Autodesk Inventor part; units mm, degrees
ref_plane "YZ Plane" through (0, 0, 0) normal (1, 0, 0) x (0, 1, 0)
ref_plane "XZ Plane" through (0, 0, 0) normal (0, 1, 0) x (-1, 0, 0)
ref_plane "XY Plane" through (0, 0, 0) normal (0, 0, 1) x (1, 0, 0)
sketch "Sketch1" plane through (0, 0, 0) normal (0, 1, 0) x (-1, 0, 0)
  line L0 (0, 0) -> (0, -40)
  line L1 (0, 0) -> (40, 0) construction
  line L2 (0, 0) -> (-60, 0)
  line L3 (-6, -40) -> (-6, -6)
  line L4 (-6, -6) -> (-60, -6)
  line L5 (-60, 0) -> (-60, -6)
  line L6 (0, -40) -> (-6, -40)
  line L7 (-60, -6) -> (-6, -40)
  dimension "d0" = 40
  dimension "d1" = 90
  dimension "d2" = 60
  dimension "d3" = 6
extrude "Extrusion1" add sketch "Sketch1" along normal blind 3
sketch "Sketch2" plane through (0, 3, 0) normal (0, 1, 0) x (1, 0, 0)
  line L0 (0, 40) -> (0, 0)
  line L1 (0, 0) -> (0, 40)
  line L2 (0, 0) -> (60, 0)
  line L3 (60, 0) -> (0, 0)
  line L4 (6, 40) -> (6, 0)
  line L5 (60, 6) -> (6, 6)
  line L6 (60, 6) -> (6, 40)
  line L7 (60, 6) -> (60, 0)
  line L8 (6, 40) -> (0, 40)
  dimension "d6" = 6
extrude "Extrusion2" add sketch "Sketch2" along normal blind 20 contours L8 L4 L2 L0 | L4 L5 L7 L2
sketch "Sketch3" plane through (6, 3, -6) normal (1, 0, 0) x (0, 0, -1)
  line L0 (34, 20) -> (-6, 20)
  line L1 (-6, 20) -> (4, 20)
  line L2 (4, 20) -> (4, 10)
  line L3 (4, 10) -> (24, 10) construction
  line L4 (4, 7) -> (24, 7)
  line L5 (24, 13) -> (4, 13)
  arc A0 (4, 13) -> (4, 7) centre (4, 10) ccw
  arc A1 (24, 7) -> (24, 13) centre (24, 10) ccw
  point P0 (-6, -3)
  point P1 (14, 10)
  dimension "d9" = 10
  dimension "d10" = 10
  dimension "d11" = 20
  dimension "d12" = 6
extrude "Extrusion3" cut sketch "Sketch3" against normal blind 20
sketch "Sketch4" plane through (60, 3, -6) normal (0, 0, -1) x (-1, 0, 0)
  line L0 (10, 20) -> (10, 10)
  line L1 (10, 10) -> (50, 10) construction
  line L2 (10, 7) -> (50, 7)
  line L3 (50, 13) -> (10, 13)
  arc A0 (10, 13) -> (10, 7) centre (10, 10) ccw
  arc A1 (50, 7) -> (50, 13) centre (50, 10) ccw
  line L4 (60, -3) -> (60, 20)
  line L5 (0, 20) -> (54, 20)
  point P0 (30, 10)
  dimension "d16" = 10
  dimension "d17" = 40
  dimension "d18" = 6
  dimension "d35" = 10
  dimension "d36" = 13
extrude "Extrusion4" cut sketch "Sketch4" against normal blind 20
fillet "Fillet1" radius 2 3 edges at (0, 11.5, 0) (60, 11.5, 0) (0, 11.5, -40)
fillet "Fillet2" radius 2 2 edges at (33, 23, -6) (6, 23, -23)
fillet "Fillet3" radius 2 11 edges at (59.4142, 23, -0.5858) (60, 23, -3) (60, 22.4142, -5.4142) (60, 12, -6) (0.5858, 23, -0.5858) (0, 23, -20) (0.5858, 23, -39.4142) (3, 23, -40) (5.4142, 22.4142, -40) (6, 12, -40) (30, 23, 0)
fillet "Fillet4" radius 2 7 edges at (0.5858, 0, -39.4142) (4, 0, -40) (0.5858, 0, -0.5858) (30, 0, 0) (59.4142, 0, -0.5858) (60, 0, -4) (0, 0, -20)
properties part number "RightAngle_Bracket_60mm"
Input: part model. Units: mm. Frame: model coordinates. A direction names the side the tool comes from. Coordinates: 2 decimals unless noted, no trailing zeros. Order: outer loops, then holes, each group sorted by start corner. A loop starts at its lowest first (then second) coordinate and runs counter-clockwise, first axis right, second up. Notation, with made-up numbers: M -18.5,38 L 32.5,38 A21 ccw 32.5,58 Z; hole C 87,39.25 d11. An arc over 180 degrees is marked long. Answer in a Markdown table with one row per item.
(1) Material intervals for line 1 (Y direction, x = 17, z = -3); line 2 (Y direction, x = 10.5, z = -18); line 3 (X direction, y = 18.5, z = -36), sorted ascending. Write a range as [from, to].
Numbers:
| item | result |
|---|---|
| line 1 | y = [0, 10], [16, 23] |
| line 2 | y = [0, 3] |
| line 3 | x = [0, 6] |
(2) Section query D-D, the plane y = 9. Output: boundary loops of the cut face in (x, z), plus the area to 3 significant figures.
Numbers:
| item | result |
|---|---|
| outline | M 0,-38 A2 ccw 2,-40 L 4,-40 A2 ccw 6,-38 L 6,-6 L 58,-6 A2 ccw 60,-4 L 60,-2 A2 ccw 58,0 L 2,0 A2 ccw 0,-2 Z |
| area | 560 mm^2 |
(3) Access query for faces 1 (the cylindrical face through (5.43, 22.4, -20.76)), 2 (the cylindrical face through (3, 13, -33)), 3 (the cylindrical face through (0.57, 11.63, -0.6)), 4 (the flat face through (30, 10, -3)). Directions: +Z, -Z, +X, -X, +Y, -Y. A direction counts if a zero-diameter tool reaches every point of the face in a straight line with its end or side. Return the directions, or none.
Numbers:
| item | result |
|---|---|
| face 1 | -Z, +X, +Y |
| face 2 | +X, -X |
| face 3 | +Z, -X, +Y, -Y |
| face 4 | +Z, -Z |
(4) Contact query for flat-ended pins moving along their axis: pin 1 Ø5 at (x, z) = (34.5, -22) entering from -Y; pin 2 Ø10 at (x, z) = (28.5, -16.5) entering from +Y; pin 3 Ø1 at (x, y) = (19.5, 19) entering from -Z. Output: stop coordinate, or through.
Numbers:
| item | result |
|---|---|
| pin 1 | stops at y = 0 |
| pin 2 | stops at y = 3 |
| pin 3 | stops at z = -6 |
(5) Section query B-B, the plane x = 28. Output: boundary loops of the cut face in (y, z).
Numbers:
| item | result |
|---|---|
| outline | M 0,-26.15 L 3,-26.15 L 3,-6 L 10,-6 L 10,0 L 2,0 A2 ccw 0,-2 Z; M 16,-6 L 21,-6 A2 ccw 23,-4 L 23,-2 A2 ccw 21,0 L 16,0 Z |
(6) Draft query along Y for faces 5 (the cylindrical face through (3, 13, -7)), 6 (the flat face through (24, 0, -16)), 7 (the cylindrical face through (5.43, 12.13, -39.4)). Return one class per face: pulls with the +Y half, pulls with the -Y half, needs draft (parallel to the pull), parting line crosses it, or undercut.
Numbers:
| item | result |
|---|---|
| face 5 | undercut |
| face 6 | pulls with the -Y half |
| face 7 | needs draft |
(7) Section query C-C, the plane z = -24.5. Output: boundary loops of the cut face in (x, y).
Numbers:
| item | result |
|---|---|
| outline | M 0,2 A2 ccw 2,0 L 30.62,0 L 30.62,3 L 6,3 L 6,10 L 0,10 Z; M 0,16 L 6,16 L 6,21 A2 ccw 4,23 L 2,23 A2 ccw 0,21 Z |
(8) Section query A-A, the plane y = 13. Output: boundary loops of the cut face in (x, z).
Numbers:
| item | result |
|---|---|
| outline | M 0,-38 A2 ccw 2,-40 L 4,-40 A2 ccw 6,-38 L 6,-33 L 0,-33 Z; M 0,-7 L 6,-7 L 6,-6 L 7,-6 L 7,0 L 2,0 A2 ccw 0,-2 Z; M 53,-6 L 58,-6 A2 ccw 60,-4 L 60,-2 A2 ccw 58,0 L 53,0 Z |
